Study the drawing (mm; zero at the part's minimum x, y, z) and answer. A direction names the side the tool comes from. Coordinates: 2 decimals unless noted, no trailing zeros. Loops run counter-clockwise (first coordinate to the right, second up) from the corner with the lowest first, then second, coordinate; pieces in that order, holes last. Notation, with made-up numbers: (-34, 62) -> (-11, 62) arc R22 cw to (-11, 97) -> close; hole circle Ø8 at (16.5, -9). An arc over 180 degrees is marked (long way). Answer in a Markdown table with one row per item.
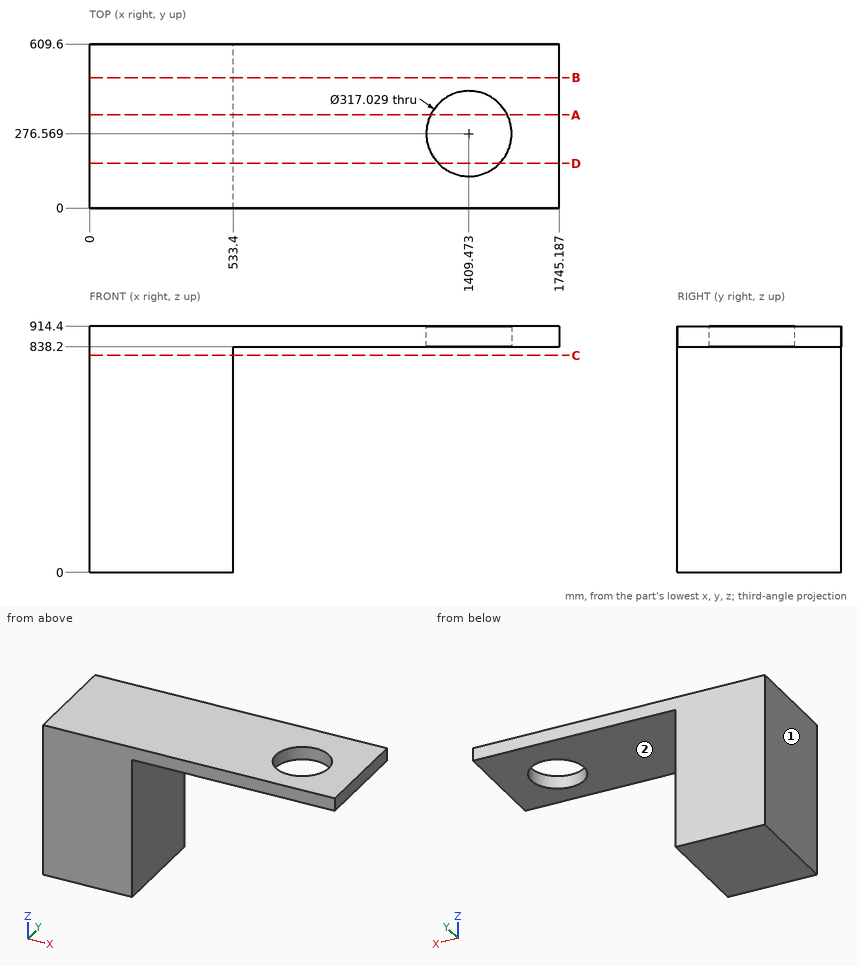
1. A cutting plane is placed at B-B on y = 485. Give the vertices of the cut face in (x, z).
A:
| item | result |
|---|---|
| outline | (0, 0) -> (533.4, 0) -> (533.4, 838.2) -> (1745.19, 838.2) -> (1745.19, 914.4) -> (0, 914.4) -> close |
2. A cutting plane is placed at C-C on z = 806. Give the vertices of the cut face in (x, y).
A:
| item | result |
|---|---|
| outline | (0, 0) -> (533.4, 0) -> (533.4, 609.6) -> (0, 609.6) -> close |
3. A cutting plane is placed at A-A on y = 346. Give the vertices of the cut face in (x, z).
A:
| item | result |
|---|---|
| outline | (0, 0) -> (533.4, 0) -> (533.4, 838.2) -> (1266.97, 838.2) -> (1266.97, 914.4) -> (0, 914.4) -> close; (1551.97, 838.2) -> (1745.19, 838.2) -> (1745.19, 914.4) -> (1551.97, 914.4) -> close |
4. A tool of negligible diameter and unlimited length cuts with its end or side. For the marked faces 1 and 2, from which of +Z, -Z, +X, -X, +Y, -Y can it reach the whole face along a straight path? Write none if from no direction.
A:
| item | result |
|---|---|
| face 1 | +Z, -Z, -X, +Y, -Y |
| face 2 | -Z, +X, +Y, -Y |
5. A cutting plane is placed at D-D on y = 166. Give the vertices of the cut face in (x, z), and give its area (3 significant figures).
A:
| item | result |
|---|---|
| outline | (0, 0) -> (533.4, 0) -> (533.4, 838.2) -> (1295.89, 838.2) -> (1295.89, 914.4) -> (0, 914.4) -> close; (1523.06, 838.2) -> (1745.19, 838.2) -> (1745.19, 914.4) -> (1523.06, 914.4) -> close |
| area | 563,000 mm2 |
6. Given pin 1 Ø4 at (y, z) = (90.5, 291.5) entering from +X; pin 2 Ø6 at (x, y) = (1125, 402) entering from -Z, each flat-ended and moving along its own axis, determine where each tip first touches the part or whether it passes through.
A:
| item | result |
|---|---|
| pin 1 | stops at x = 533.4 |
| pin 2 | stops at z = 838.2 |
7. Find the intervals of material crossed by probe 1 along Z at (x, y) = (703.5, 532.5); probe 2 along X at (y, z) = (429, 668.5), in increasing order.
A:
| item | result |
|---|---|
| probe 1 | z = 838.2 to 914.4 |
| probe 2 | x = 0 to 533.4 |
